Here's the drawing with two shaded views (mm, measured from the low corner). I have some questions. A direction names the side the tool comes from. Coordinates: 2 decimals unless noted, no trailing zeros. Write each loop counter-clockwise with the first axis right and the second up, starting at its lowest first coordinate (ties: lowest second). Pieces come first, ordered by that corner, then holes. Notation, with made-up numbers: (-22.5, 61.25) -> (35.5, 61.25) arc R9 cw to (35.5, 71.25) -> close; hole circle Ø9 at (-14, 43). An arc over 180 degrees is marked (long way). Put each result on its own line as item: value.
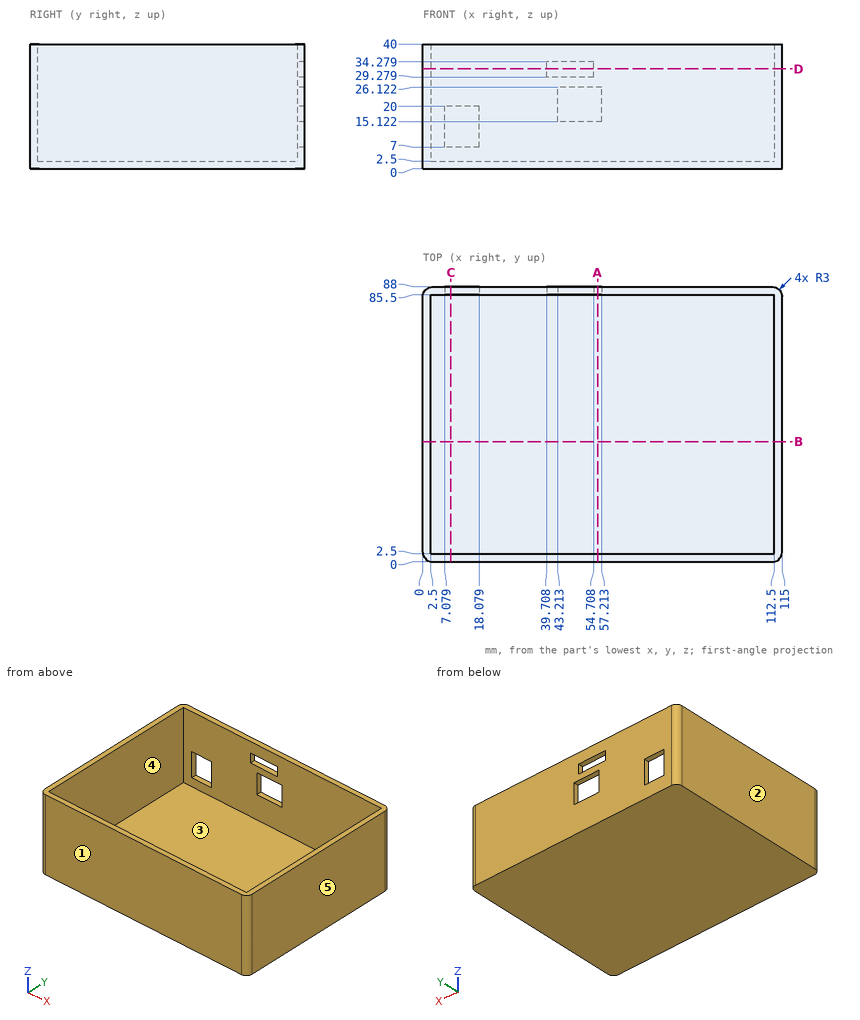
Item 1: Imagine slicing it at B-B on y = 38.5. Write out the boundary of the cut face in (x, z), then the cut area to 3 significant figures.
Output:
outline: (0, 0) -> (115, 0) -> (115, 40) -> (112.5, 40) -> (112.5, 2.5) -> (2.5, 2.5) -> (2.5, 40) -> (0, 40) -> close
area: 475 mm²
Item 2: Imagine slicing it at A-A on x = 56. Write out the boundary of the cut face in (y, z).
Output:
outline: (0, 0) -> (88, 0) -> (88, 15.12) -> (85.5, 15.12) -> (85.5, 2.5) -> (2.5, 2.5) -> (2.5, 40) -> (0, 40) -> close; (85.5, 26.12) -> (88, 26.12) -> (88, 40) -> (85.5, 40) -> close
Item 3: For P1, Ø2, axis at y = 87, z = 13, coming from the -X side; P2, Ø2, axis at x = 78.5, y = 78, coming from the +Z side; P3, Ø3, axis at y = 87, z = 22, coming from the +X side, each with a flat end and sliding along its axis, tell me the tip position at first contact or that it passes through.
Output:
P1: stops at x = 0.17
P2: stops at z = 2.5
P3: stops at x = 114.96
Item 4: Imagine slicing it at C-C on x = 9. Write out the boundary of the cut face in (y, z), then the cut area to 3 significant figures.
Output:
outline: (0, 0) -> (88, 0) -> (88, 7) -> (85.5, 7) -> (85.5, 2.5) -> (2.5, 2.5) -> (2.5, 40) -> (0, 40) -> close; (85.5, 20) -> (88, 20) -> (88, 40) -> (85.5, 40) -> close
area: 375 mm²
Item 5: Please list where these lines run through material, in increasing order: line 1 along Y through (x, z) = (80, 38); line 2 along X through (y, z) = (37.5, 9); line 3 along Z through (x, y) = (18, 30). Write a range as from..to.
Output:
line 1: y = 0..2.5, 85.5..88
line 2: x = 0..2.5, 112.5..115
line 3: z = 0..2.5
Item 6: Which directions (+Z, -Z, +X, -X, +Y, -Y) give clear straight access to the entire face, cutting with the end or side of a thin tool? Please do the marked faces 4 and 5.
Output:
face 4: +Z
face 5: +Z, -Z, +X, +Y, -Y
Item 7: If we mould it in two halves opening along Y, with no side actions, what happens to the marked faces 1, 2 and 3? For each: released by +Y, released by -Y, zero draft, split by the parting line, or undercut.
Output:
face 1: released by -Y
face 2: zero draft
face 3: undercut
Item 8: Imagine slicing it at D-D on z = 32. Write out the boundary of the cut face in (x, y).
Output:
outline: (0, 3) arc R3 ccw to (3, 0) -> (112, 0) arc R3 ccw to (115, 3) -> (115, 85) arc R3 ccw to (112, 88) -> (54.71, 88) -> (54.71, 85.5) -> (112.5, 85.5) -> (112.5, 2.5) -> (2.5, 2.5) -> (2.5, 85.5) -> (39.71, 85.5) -> (39.71, 88) -> (3, 88) arc R3 ccw to (0, 85) -> close
